from build123d import *

# Parameters (mm, degrees)
EXTRUDE_2_DEPTH = 9
SKETCH_3_W      = 860
SKETCH_3_H      = 16
EXTRUDE_3_DEPTH = 70
SKETCH_4_W      = 140
SKETCH_4_H      = 50
EXTRUDE_5_DEPTH = 11
SKETCH_6_W      = 140
SKETCH_6_H      = 50
EXTRUDE_6_DEPTH = 6
SKETCH_10_W     = 429
SKETCH_10_H     = 16
EXTRUDE_8_DEPTH = 79


with BuildPart() as part:
    # 草图1 → 凸台-拉伸2 (new body)
    with BuildSketch(Plane.XY):
        Polygon((0, 0), (860, 0), (860, 16), (804.5, 16), (804.5, 290), (724.5, 290), (644.5, 210), (644.5, 226), (215.5, 226), (215.5, 210), (135.5, 290), (55.5, 290), (55.5, 16), (0, 16), align=None)
    extrude(amount=EXTRUDE_2_DEPTH)

    # 草图3 → 凸台-拉伸3 (add)
    with BuildSketch(Plane.XY.offset(9)):
        with Locations((430, 8)):
            Rectangle(SKETCH_3_W, SKETCH_3_H)
    extrude(amount=EXTRUDE_3_DEPTH)

    # 草图4 → 凸台-拉伸5 (add)
    with BuildSketch(Plane(origin=(0, 16, 0), x_dir=(1, 0, 0), z_dir=(0, 1, 0))):
        with Locations((90, -48)):
            Rectangle(SKETCH_4_W, SKETCH_4_H)
    extrude(amount=EXTRUDE_5_DEPTH)

    # 草图6 → 凸台-拉伸6 (add)
    with BuildSketch(Plane(origin=(0, 16, 0), x_dir=(1, 0, 0), z_dir=(0, 1, 0))):
        with Locations((770, -48)):
            Rectangle(SKETCH_6_W, SKETCH_6_H)
    extrude(amount=EXTRUDE_6_DEPTH)

    # 草图10 → 凸台-拉伸8 (add)
    with BuildSketch(Plane.XY.offset(9)):
        with Locations((430, 218)):
            Rectangle(SKETCH_10_W, SKETCH_10_H)
    extrude(amount=EXTRUDE_8_DEPTH)


solid = part.part
Geometry check sheet. Reference: the model listing, model coordinates, mm. A direction names the side the tool comes from. Give positions to 0.01 mm unless a question says otherwise; leave off trailing zeros. Order: outer loops, then holes, each group sorted by start corner. A loop starts at its lowest first (then second) coordinate and runs counter-clockwise, first axis right, second up. Notation, with made-up numbers: M 19.5,35.25 L 45.5,35.25 A19 cw 45.5,58.25 Z; hole C 1,-20.75 d8. An arc over 180 degrees is marked long. Use a Markdown table: item, result.
Item 1: Section check C-C (x = 503.5). Record the cut outline in (y, z), and give its area (3 significant figures).
Answers follow:
| item | result |
|---|---|
| outline | M 0,0 L 226,0 L 226,88 L 210,88 L 210,9 L 16,9 L 16,79 L 0,79 Z |
| area | 4,420 mm2 |
Item 2: Material ranges on line 1 along Y through (x, z) = (427, 19.5); line 2 along Y through (x, z) = (100.5, 55.5); line 3 along Z through (x, y) = (218.5, 187.5), recorded low to high.
Answers follow:
| item | result |
|---|---|
| line 1 | y = 0 to 16, 210 to 226 |
| line 2 | y = 0 to 27 |
| line 3 | z = 0 to 9 |
Item 3: Section check D-D (x = 77.5). Record the cut outline in (y, z), and give its area (3 significant figures).
Answers follow:
| item | result |
|---|---|
| outline | M 0,0 L 290,0 L 290,9 L 16,9 L 16,23 L 27,23 L 27,73 L 16,73 L 16,79 L 0,79 Z |
| area | 4,280 mm2 |
Item 4: Section check B-B (y = 254). Record the cut outline in (x, z).
Answers follow:
| item | result |
|---|---|
| outline | M 55.5,0 L 171.5,0 L 171.5,9 L 55.5,9 Z; M 688.5,0 L 804.5,0 L 804.5,9 L 688.5,9 Z |
Item 5: Tool access check on faces 1 (the flat face through (685.1, 250.6, 4.4)), 2 (the flat face through (427, 210, 48)), 3 (the flat face through (89, 27, 48)), 4 (the flat face through (769, 22, 48)), 5 (the flat face through (424, 0, 39)). Record the directions out of +Z, -Z, +X, -X, +Y, -Y that give a thin tool (end or side, any length) a straight path to the whole face; none if there is none.
Answers follow:
| item | result |
|---|---|
| face 1 | +Z, -Z, +Y |
| face 2 | +Z, +X, -X |
| face 3 | +Z, +X, -X, +Y |
| face 4 | +Z, +X, +Y |
| face 5 | +Z, -Z, +X, -X, -Y |
Item 6: Section check A-A (z = 47). Record the cut outline in (x, y), and give its area (3 significant figures).
Answers follow:
| item | result |
|---|---|
| outline | M 0,0 L 860,0 L 860,16 L 840,16 L 840,22 L 700,22 L 700,16 L 160,16 L 160,27 L 20,27 L 20,16 L 0,16 Z; M 215.5,210 L 644.5,210 L 644.5,226 L 215.5,226 Z |
| area | 23,000 mm2 |
Item 7: Draft check along Y on faces 6 (the flat face through (425, 124, 9)), 7 (the flat face through (424, 16, 39)), 8 (the flat face through (424, 8, 79)), 9 (the flat face through (176.1, 249.4, 4.4)). Enter one of: +Y half, -Y half, draft (parallel to the pull), parting line (faces both ways), or undercut.
Answers follow:
| item | result |
|---|---|
| face 6 | undercut |
| face 7 | undercut |
| face 8 | draft |
| face 9 | +Y half |
Item 8: Depth check by flat-ended pin: P1, Ø13, axis at y = 214.5, z = 58, coming from the +X side; P2, Ø4, axis at x = 253, y = 143, coming from the +Z side; P3, Ø8, axis at y = 242, z = 12.5, coming from the -X side. Enter the tip coordinate at first touch or a pass-through.
Answers follow:
| item | result |
|---|---|
| P1 | stops at x = 644.5 |
| P2 | stops at z = 9 |
| P3 | stops at x = 55.5 |
